from build123d import *

# Parameters (mm, degrees)
SKETCH_1_W      = 90
SKETCH_1_H      = 28.115702479
EXTRUDE_1_DEPTH = 10
SKETCH_2_W      = 20.999219252
SKETCH_2_H      = 12.492407229
EXTRUDE_2_DEPTH = 30
SKETCH_3_W      = 5
SKETCH_3_H      = 28.115702479
EXTRUDE_3_DEPTH = 30


with BuildPart() as part:
    # 草图1 → 凸台-拉伸1 (new body)
    with BuildSketch(Plane.XY):
        with Locations((2.674645003, 3.474778593)):
            Rectangle(SKETCH_1_W, SKETCH_1_H)
    extrude(amount=EXTRUDE_1_DEPTH)

    # 草图2 → 凸台-拉伸2 (add)
    with BuildSketch(Plane.XY.offset(10)):
        with Locations((0, 3.474778592)):
            Rectangle(SKETCH_2_W, SKETCH_2_H)
    extrude(amount=EXTRUDE_2_DEPTH)

    # 草图3 → 凸台-拉伸3 (add)
    with BuildSketch(Plane(origin=(0, 0, 0), x_dir=(-1, 0, 0), z_dir=(0, 0, -1))):
        with Locations((39.825354997, 3.474778593)):
            Rectangle(SKETCH_3_W, SKETCH_3_H)
        with Locations((-45.174645003, 3.474778593)):
            Rectangle(SKETCH_3_W, SKETCH_3_H)
    extrude(amount=EXTRUDE_3_DEPTH)


solid = part.part
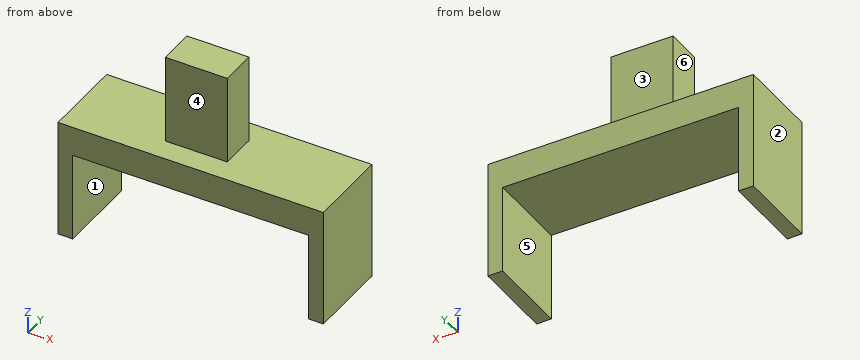
Check sheet for the modelled part. Datum: model origin and axes. Units: mm. Face numbers are marked on the shaded views. A direction names the side the tool comes from. Give positions to 0.01 mm unless a question says otherwise; leave off trailing zeros. Loops run counter-clockwise (first coordinate to the right, second up) from the corner with the lowest first, then second, coordinate; pieces in that order, holes last. Notation, with made-up numbers: M 26.25,83.5 L 72.25,83.5 A22 ccw 72.25,96.5 Z; hole C -8.75,1 d7. An arc over 180 degrees is marked long. Answer as a JSON object with one key per item and string values. Group by question number.
Q1. Cross-section at B-B on y = -7.5. Record the cut outline in (x, z), then the cut area to 3 significant figures.
Q2. Cross-section at C-C on z = 26. Record the cut outline in (x, y).
Q3. Go/stop test with flat-tipped pins: P1, Ø3.5, axis at y = 2.5, z = 29, coming from the +X side; P2, Ø6.5, axis at x = 5, z = 28, coming from the -Y side; P3, Ø1, axis at x = -20, y = 5.5, coming from the -Z side. Record where each tip stops, or that it passes through.
Q4. Access from +Z, -Z, +X, -X, +Y, -Y to the whole of each face (thin tool, end or side, straight path). Record for the marked faces 4, 5 and 6.
Q5. Cross-section at D-D on y = 0.5. Record the cut outline in (x, z), then the cut area to 3 significant figures.
Q6. Cross-section at A-A on x = -5. Record the cut outline in (y, z).
Q7. Release check for a two-part mould opening along X. For the marked faces 1, 2 and 3 record: released by +X, released by -X, zero draft, split by the parting line, or undercut.
Q8. Material ranges on line 1 along X through (y, z) = (0, -17); line 2 along Z through (x, y) = (38.5, -6); line 3 along Z through (x, y) = (-8, -1.5), recorded low to high. Write a range as [from, to].
Evaluation:
{
 "1": {"outline": "M -42.33,-30 L -37.33,-30 L -37.33,0 L 42.67,0 L 42.67,-30 L 47.67,-30 L 47.67,10 L -42.33,10 Z", "area": "1,200 mm2"},
 "2": {"outline": "M -10.5,-2.77 L 10.5,-2.77 L 10.5,9.72 L -10.5,9.72 Z"},
 "3": {"P1": "stops at x = 10.5", "P2": "stops at y = -2.77", "P3": "stops at z = 0"},
 "4": {"face 4": "+Z, +X, -X, -Y", "face 5": "-Z, +Y, -Y", "face 6": "+Z, -X, +Y, -Y"},
 "5": {"outline": "M -42.33,-30 L -37.33,-30 L -37.33,0 L 42.67,0 L 42.67,-30 L 47.67,-30 L 47.67,10 L 10.5,10 L 10.5,40 L -10.5,40 L -10.5,10 L -42.33,10 Z", "area": "1,830 mm2"},
 "6": {"outline": "M -10.58,0 L 17.53,0 L 17.53,10 L 9.72,10 L 9.72,40 L -2.77,40 L -2.77,10 L -10.58,10 Z"},
 "7": {"face 1": "undercut", "face 2": "released by -X", "face 3": "zero draft"},
 "8": {"line 1": "x = [-42.33, -37.33], [42.67, 47.67]", "line 2": "z = [0, 10]", "line 3": "z = [0, 40]"}
}
